from build123d import *

# Parameters (mm, degrees)
AUFSATZ_LINEAR_AUSTRAGEN1_DEPTH      = 5
F_8_6_8_6_DURCHMESSER_BOHRUNG1_D     = 8.6
F_8_6_8_6_DURCHMESSER_BOHRUNG1_DEPTH = 80
F_8_6_8_6_DURCHMESSER_BOHRUNG1_TIP   = 2.583700662
FASE1_SIZE                           = 4
FASE1_SIZE2                          = 14.92820323


with BuildPart() as part:
    # Skizze1 → Aufsatz-Linear austragen1 (new body)
    with BuildSketch(Plane.XY):
        Polygon((-34, 50), (-22, 62), (22, 62), (34, 50), (34, 0), (-34, 0), align=None)
    extrude(amount=AUFSATZ_LINEAR_AUSTRAGEN1_DEPTH)

    # Ø8.6 (8.6) Durchmesser Bohrung1
    with Locations(Plane.XY.offset(5)):
        with Locations((0, 45)):
            Hole(F_8_6_8_6_DURCHMESSER_BOHRUNG1_D / 2, depth=F_8_6_8_6_DURCHMESSER_BOHRUNG1_DEPTH)
            with Locations((0, 0, -(F_8_6_8_6_DURCHMESSER_BOHRUNG1_DEPTH + F_8_6_8_6_DURCHMESSER_BOHRUNG1_TIP / 2))):  # 118° drill point
                Cone(0, F_8_6_8_6_DURCHMESSER_BOHRUNG1_D / 2, F_8_6_8_6_DURCHMESSER_BOHRUNG1_TIP, mode=Mode.SUBTRACT)

    # Fase1
    fase1_edges = [part.edges().sort_by_distance(p)[0] for p in [
        (0, 0, 5),
    ]]
    fase1_side = [part.faces().sort_by_distance(p)[0] for p in [
        (0, 0, 2.5),
    ]]
    chamfer(fase1_edges, length=FASE1_SIZE, length2=FASE1_SIZE2, reference=fase1_side[0])


solid = part.part
Geometry check sheet. Reference: the model listing, model coordinates, mm. Give positions to 0.01 mm unless a question says otherwise; leave off trailing zeros. Order: outer loops, then holes, each group sorted by start corner. A loop starts at its lowest first (then second) coordinate and runs counter-clockwise, first axis right, second up. Notation, with made-up numbers: (12, 64.5) - (37, 64.5) arc R20 cw to (37, 70.5) - close; hole circle Ø3 at (-14.5, -34.5). An arc over 180 degrees is marked (long way). Use one line per item in the form item = value.
1) Material ranges on probe 1 along X at (y, z) = (44, 2.6); probe 2 along X at (y, z) = (41.5, 2.5); probe 3 along Z at (x, y) = (15.5, 11.5), recorded low to high. Write a range as from..to.
Working result:
probe_1 = -34..-4.18, 4.18..34
probe_2 = -34..-2.5, 2.5..34
probe_3 = 0..4.08
2) Sectioned sample at C-C (z = 2.1). Record the boundary of the cut face in (x, y), and give its area (3 significant figures).
Working result:
outline = (-34, 4.11) - (34, 4.11) - (34, 50) - (22, 62) - (-22, 62) - (-34, 50) - close; hole circle Ø8.6 at (0, 45)
area = 3,730 mm^2
3) Draft check along X on faces 1 (the face through (0.93, 40.8, 2.47)), 2 (the face through (34, 25, 2)), 3 (the face through (0, 62, 2)). Enter one of: released by +X, released by -X, zero draft, split by the parting line, or undercut.
Working result:
face_1 = undercut
face_2 = released by +X
face_3 = zero draft
4) Sectioned sample at A-A (x = 0). Record the boundary of the cut face in (y, z).
Working result:
outline = (0, 0) - (40.7, 0) - (40.7, 5) - (14.93, 5) - (0, 1) - close; (49.3, 0) - (62, 0) - (62, 5) - (49.3, 5) - close
5) Depth check by flat-ended pin: pin 1 Ø1.5 at (x, y) = (-2, 7.5) entering from +Z. Enter the tip coordinate at first touch or a pass-through.
Working result:
pin_1 = 3.21
6) Sectioned sample at B-B (y = 45). Record the boundary of the cut face in (x, z).
Working result:
outline = (-34, 0) - (-4.3, 0) - (-4.3, 5) - (-34, 5) - close; (4.3, 0) - (34, 0) - (34, 5) - (4.3, 5) - close
7) Sectioned sample at D-D (x = 15). Record the boundary of the cut face in (y, z).
Working result:
outline = (0, 0) - (62, 0) - (62, 5) - (14.93, 5) - (0, 1) - close
